from build123d import *

# Parameters (mm, degrees)
SKETCH3_R                    = 200
BASE_FLANGE1_DEPTH           = 3
F_30_0_1285_DIAMETER_HOLE1_D = 3.2639


# Sheet-metal steps are written as plain solids
with BuildPart() as part:
    # Sketch3 → Base-Flange1 (new body)
    with BuildSketch(Plane(origin=(0, 0, 0), x_dir=(1, 0, 0), z_dir=(0, 1, 0))):
        with Locations(Location((0, 0, 0), (0, 0, 270))):
            Circle(SKETCH3_R)
    extrude(amount=-BASE_FLANGE1_DEPTH)

    # #30 (0.1285) Diameter Hole1 (through all)
    with Locations(Plane(origin=(0, 0, 0), x_dir=(1, 0, 0), z_dir=(0, 1, 0))):
        with Locations((0, 150), (0, 100), (0, 50), (50, 0), (100, 0), (150, 0), (0, -50), (0, -100), (0, -150), (-50, 0), (-100, 0), (-150, 0)):
            Hole(F_30_0_1285_DIAMETER_HOLE1_D / 2)


solid = part.part
Could you check a few things on this model? Use its own coordinates, in mm. Coordinates: 2 decimals unless noted, no trailing zeros. Order: outer loops, then holes, each group sorted by start corner. A loop starts at its lowest first (then second) coordinate and runs counter-clockwise, first axis right, second up.
Q1. Will these pins go through, and if not, where does the flat tip stop? pin 1 (2 mm diameter, centred on x = -50, z = 0, fed in from +Y); pin 2 (1 mm diameter, centred on y = -0.5, z = 105, fed in from -X).
Q2. Please list where these lines run through material, in increasing order: L1, parallel to Z at x = -134, y = -0.95; L2, parallel to Z at x = 50, y = -1.6; L3, parallel to X at y = -1.8, z = 132.
Q3. Suppose I cut it at B-B on x = 127. Please give me the cut outline in (y, z).
Q4. Suppose I cut it at C-C on z = -106.5. Please give me the cut outline in (x, y).
Q5. Suppose I cut it at A-A on y = -1.65. Give the number of separate pieces and of enclosed holes in the cut face, and give its area (3 significant figures).
Answer:
1. pin 1: passes through
1. pin 2: stops at x = -170.53
2. L1: z = -148.47 to 148.47
2. L2: z = -193.65 to -1.63, 1.63 to 193.65
2. L3: x = -150.25 to 150.25
3. outline: (-3, -154.5) - (0, -154.5) - (0, 154.5) - (-3, 154.5) - close
4. outline: (-169.29, -3) - (169.29, -3) - (169.29, 0) - (-169.29, 0) - close
5. separate pieces: 1
5. enclosed holes: 12
5. area: 126,000 mm2
